Source: CAD feature listing. Evaluate the final solid. Frame: model axes, mm. A direction names the side the tool comes from. Give positions to 0.01 mm unless a question says otherwise; leave off trailing zeros. Order: outer loops, then holes, each group sorted by start corner. A loop starts at its lowest first (then second) coordinate and runs counter-clockwise, first axis right, second up. Notation, with made-up numbers: M 78.5,9 L 106.5,9 A30 cw 106.5,47 Z; hole C 3.5,61 d10. An arc over 180 degrees is marked long. Answer as a JSON object with one key per item and string values. Group by question number.
1. Section query A-A (z = -4). Count the separate pieces of the cut face and the enclosed holes in it, plus the area to 3 significant figures.
2. Pin query (flat end, axial travel): P1, Ø4.5, axis at x = 96.5, y = -4, coming from the -Z side; P2, Ø10, axis at x = 31, y = -21, coming from the +Z side; P3, Ø3.5, axis at x = 97, z = -19, coming from the +Y side; P4, Ø1, axis at y = -18, z = -7.5, coming from the +X side. Return the tip coordinate at first contact, or that it passes through.
3. Pull-direction query (Y, two-part tool) for faces 1 (the cylindrical face through (94, -20, -2)), 2 (the flat face through (78, -26, -14)), 3 (the flat face through (22, -27, -2.5)); classes: +Y half, -Y half, draft (parallel to the pull), parting line (faces both ways), or undercut.
4. Section query C-C (x = 52.5). Output: boundary loops of the cut face in (y, z), plus the area to 3 significant figures.
5. Material intervals for L1, parallel to Y at x = 96.5, z = -1.7; L2, parallel to X at y = -22, z = -24.5; L3, parallel to Y at x = 96, z = -3, sorted ascending. Write a range as [from, to].
6. Section query B-B (x = 3.5). Output: boundary loops of the cut face in (y, z), plus the area to 3 significant figures.
7. Set-up query: faces 4 (the flat face through (5, -15, 0)), 5 (the flat face through (22, -26, -14)), 6 (the flat face through (7, -13, -17)). Return all of +Z, -Z, +X, -X, +Y, -Y with unobstructed straight access to the full face (end or side cutting, diameter ignored); none if empty.
from build123d import *

# Parameters (mm, degrees)
SKETCH3_W           = 100
SKETCH3_H           = 30
BOSS_EXTRUDE1_DEPTH = 30
SKETCH3_6_R         = 2.5
CUT_EXTRUDE1_DEPTH  = 25
CUT_EXTRUDE2_DEPTH  = 5
CUT_EXTRUDE3_START  = -5
SKETCH3_9_W         = 7
SKETCH3_9_H         = 26
SKETCH3_9_R         = 2.5
CUT_EXTRUDE3_DEPTH  = 104.627804912
CUT_EXTRUDE4_DEPTH  = 2.5
BOSS_EXTRUDE2_DEPTH = 2.5


with BuildPart() as part:
    # Sketch3 → Boss-Extrude1 (new body)
    with BuildSketch(Plane.XY):
        with Locations((50, -15)):
            Rectangle(SKETCH3_W, SKETCH3_H)
    extrude(amount=-BOSS_EXTRUDE1_DEPTH)

    # Sketch3_6 → Cut-Extrude1 (cut)
    with BuildSketch(Plane.XY):
        Polygon((35.214289751, 0), (8.952376915, 0), (9.860316922, -26), (34.306349745, -26), align=None)
        Polygon((61.880956418, 0), (38.119043582, 0), (39.026983589, -26), (60.973016411, -26), align=None)
        Polygon((91.047623085, 0), (64.785710249, 0), (65.693650255, -26), (90.139683078, -26), align=None)
        with Locations((3.5, -4)):
            Circle(SKETCH3_6_R)
        with Locations((3.5, -12)):
            Circle(SKETCH3_6_R)
        with Locations((3.5, -20)):
            Circle(SKETCH3_6_R)
        with Locations((96.5, -12)):
            Circle(SKETCH3_6_R)
        with Locations((96.5, -4)):
            Circle(SKETCH3_6_R)
        with Locations((96.5, -20)):
            Circle(SKETCH3_6_R)
    extrude(amount=-CUT_EXTRUDE1_DEPTH, mode=Mode.SUBTRACT)

    # Sketch3_8 → Cut-Extrude2 (cut)
    with BuildSketch(Plane.XY):
        Polygon((37.118434038, 0), (36.214899296, 0), (35.306959289, -26), (38.026374044, -26), align=None)
        Polygon((63.785100704, 0), (62.881565962, 0), (61.973625956, -26), (64.693040711, -26), align=None)
        Polygon((38.026374044, -26), (35.306959289, -26), (35.23711775, -28), (38.096215583, -28), align=None)
        Polygon((38.096215583, -28), (35.23711775, -28), (35.167276211, -30), (38.166057122, -30), align=None)
        Polygon((64.693040711, -26), (61.973625956, -26), (61.903784417, -28), (64.76288225, -28), align=None)
        Polygon((64.76288225, -28), (61.903784417, -28), (61.833942878, -30), (64.832723789, -30), align=None)
    extrude(amount=-CUT_EXTRUDE2_DEPTH, mode=Mode.SUBTRACT)

    # Sketch3_9 → Cut-Extrude3 (cut, through all)
    # profile 1 of 8: a face of its own
    with BuildSketch(Plane.XY.offset(CUT_EXTRUDE3_START)):
        with Locations((3.5, -13)):
            Rectangle(SKETCH3_9_W, SKETCH3_9_H)
        with Locations((3.5, -20)):
            Circle(SKETCH3_9_R, mode=Mode.SUBTRACT)
        with Locations((3.5, -12)):
            Circle(SKETCH3_9_R, mode=Mode.SUBTRACT)
        with Locations((3.5, -4)):
            Circle(SKETCH3_9_R, mode=Mode.SUBTRACT)
    # profile 2 of 8: a face of its own
    with BuildSketch(Plane.XY.offset(CUT_EXTRUDE3_START)):
        with Locations((96.5, -13)):
            Rectangle(SKETCH3_9_W, SKETCH3_9_H)
        with Locations((96.5, -20)):
            Circle(SKETCH3_9_R, mode=Mode.SUBTRACT)
        with Locations((96.5, -12)):
            Circle(SKETCH3_9_R, mode=Mode.SUBTRACT)
        with Locations((96.5, -4)):
            Circle(SKETCH3_9_R, mode=Mode.SUBTRACT)
    # profile 3 of 8: a face of its own
    with BuildSketch(Plane.XY.offset(CUT_EXTRUDE3_START)):
        with Locations((3.5, -4)):
            Circle(SKETCH3_9_R)
    # profile 4 of 8: a face of its own
    with BuildSketch(Plane.XY.offset(CUT_EXTRUDE3_START)):
        with Locations((3.5, -12)):
            Circle(SKETCH3_9_R)
    # profile 5 of 8: a face of its own
    with BuildSketch(Plane.XY.offset(CUT_EXTRUDE3_START)):
        with Locations((3.5, -20)):
            Circle(SKETCH3_9_R)
    # profile 6 of 8: a face of its own
    with BuildSketch(Plane.XY.offset(CUT_EXTRUDE3_START)):
        with Locations((96.5, -20)):
            Circle(SKETCH3_9_R)
    # profile 7 of 8: a face of its own
    with BuildSketch(Plane.XY.offset(CUT_EXTRUDE3_START)):
        with Locations((96.5, -4)):
            Circle(SKETCH3_9_R)
    # profile 8 of 8: a face of its own
    with BuildSketch(Plane.XY.offset(CUT_EXTRUDE3_START)):
        with Locations((96.5, -12)):
            Circle(SKETCH3_9_R)
    extrude(amount=-CUT_EXTRUDE3_DEPTH, mode=Mode.SUBTRACT)

    # Sketch3_10 → Cut-Extrude4 (cut)
    with BuildSketch(Plane.XY):
        Polygon((34.306349745, -26), (9.860316922, -26), (9.930158461, -28), (34.236508206, -28), align=None)
        Polygon((60.973016411, -26), (39.026983589, -26), (39.096825128, -28), (60.903174872, -28), align=None)
        Polygon((90.139683078, -26), (65.693650255, -26), (65.763491794, -28), (90.069841539, -28), align=None)
    extrude(amount=-CUT_EXTRUDE4_DEPTH, mode=Mode.SUBTRACT)

    # Sketch3_11 → Boss-Extrude2 (add)
    with BuildSketch(Plane.XY):
        Polygon((34.236508206, -28), (9.930158461, -28), (10, -30), (34.166666667, -30), align=None)
        Polygon((60.903174872, -28), (39.096825128, -28), (39.166666667, -30), (60.833333333, -30), align=None)
        Polygon((90.069841539, -28), (65.763491794, -28), (65.833333333, -30), (90, -30), align=None)
    extrude(amount=BOSS_EXTRUDE2_DEPTH)


solid = part.part
Answer sheet:
{
 "1": {"separate pieces": "3", "enclosed holes": "6", "area": "853 mm^2"},
 "2": {"P1": "through", "P2": "z = 0", "P3": "y = -26", "P4": "x = 93"},
 "3": {"face 1": "undercut", "face 2": "+Y half", "face 3": "draft"},
 "4": {"outline": "M -30,-30 L 0,-30 L 0,-25 L -26,-25 L -26,-2.5 L -28,-2.5 L -28,2.5 L -30,2.5 Z", "area": "250 mm^2"},
 "5": {"L1": "[-30, -22.5], [-17.5, -14.5], [-9.5, -6.5], [-1.5, 0]", "L2": "[7, 9.72], [34.45, 38.89], [61.11, 65.55], [90.28, 93]", "L3": "[-30, -22.45], [-17.55, -14.45], [-9.55, -6.45], [-1.55, 0]"},
 "6": {"outline": "M -30,-30 L -26,-30 L -26,-5 L -22.5,-5 L -22.5,0 L -30,0 Z; M -17.5,-5 L -14.5,-5 L -14.5,0 L -17.5,0 Z; M -9.5,-5 L -6.5,-5 L -6.5,0 L -9.5,0 Z; M -1.5,-5 L 0,-5 L 0,0 L -1.5,0 Z", "area": "175 mm^2"},
 "7": {"face 4": "+Z, -X, +Y, -Y", "face 5": "+Z, +Y", "face 6": "-Z, -X, +Y"}
}
